Check sheet for the modelled part. Datum: model origin and axes. Units: mm. Face numbers are marked on the shaded views. Round coordinates to 2 decimals unless told otherwise and drop trailing zeros. Order: outer loops, then holes, each group sorted by start corner. A loop starts at its lowest first (then second) coordinate and runs counter-clockwise, first axis right, second up. Notation, with made-up numbers: (22.25, 29.25) -> (46.25, 29.25) arc R22 cw to (46.25, 52.25) -> close; hole circle Ø1 at (-40, 83.5). An arc over 180 degrees is marked (long way). Use CSV: the item, a comma, the result in double quotes.
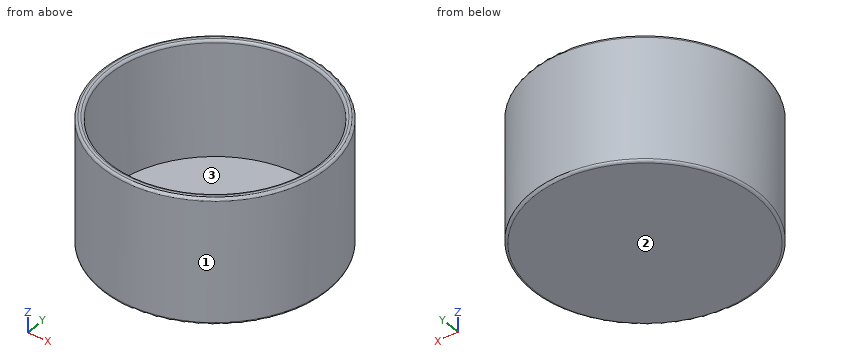
```python
from build123d import *

# Parameters (mm, degrees)
F0_R     = 57.15
F1_DEPTH = 5.08
F2_R     = 1.27
F5_E1_W  = 63.5
F5_E1_H  = 3.81
F7_R     = 1.26999
F8_R     = 1.27


# Not quite as in the source:
# - a fillet or chamfer is up to 0.001 mm smaller than in the source, because OpenCascade refuses the exact size


with BuildPart() as f1:
    # F0 (on Top) → F1 (new body)
    with BuildSketch(Plane.XY):
        Circle(F0_R)
    extrude(amount=F1_DEPTH)

    # F2
    f2_edges = [f1.edges().sort_by_distance(p)[0] for p in [
        (-57.15, 0, 0),
    ]]
    fillet(f2_edges, radius=F2_R)

    # F5_E1 (on explicit) → F6 (revolve)
    with BuildSketch(Plane(origin=(57.15, 0, 0), x_dir=(0, 0, 1), z_dir=(0, -1, 0))):
        with Locations((31.75, 1.905)):
            Rectangle(F5_E1_W, F5_E1_H)
    revolve(axis=Axis((0, 0, 5.08), (0, 0, 1)))

    # F7 (radius 1.27 in the source; OpenCascade refuses exactly that, so slightly less here)
    f7_edges = [f1.edges().sort_by_distance(p)[0] for p in [
        (-57.15, 0, 0),
    ]]
    fillet(f7_edges, radius=F7_R)

    # F8
    f8_edges = [f1.edges().sort_by_distance(p)[0] for p in [
        (-57.15, 0, 63.5),
        (-53.34, 0, 63.5),
    ]]
    fillet(f8_edges, radius=F8_R)


solid = f1.part
```
Q1. Mould release check, pull along Y, two halves, no side actions. Record for the marked faces 1, 2 and 3: pulls with the +Y half, pulls with the -Y half, needs draft (parallel to the pull), parting line crosses it, or undercut.
Result sheet:
face 1,"parting line crosses it"
face 2,"needs draft"
face 3,"undercut"
Q2. Sectioned sample at A-A, the plane y = 0. Enter the section's corners in (x, z), then the cut area to 3 significant figures.
Result sheet:
outline,"(-57.15, 1.27) arc R1.27 ccw to (-55.88, 0) -> (55.88, 0) arc R1.27 ccw to (57.15, 1.27) -> (57.15, 62.23) arc R1.27 ccw to (55.88, 63.5) -> (54.61, 63.5) arc R1.27 ccw to (53.34, 62.23) -> (53.34, 5.08) -> (-53.34, 5.08) -> (-53.34, 62.23) arc R1.27 ccw to (-54.61, 63.5) -> (-55.88, 63.5) arc R1.27 ccw to (-57.15, 62.23) -> close"
area,"1,020 mm^2"
Q3. Sectioned sample at C-C, the plane z = 44. Enter the section's corners in (x, y).
Result sheet:
outline,"circle Ø114.3 at (0, 0); hole circle Ø106.68 at (0, 0)"
Q4. Go/stop test with flat-tipped pins: pin 1 (1.5 mm diameter, centred on x = -15.5, z = 43, fed in from -Y); pin 2 (2 mm diameter, centred on y = 25.5, z = 55.5, fed in from -X); pin 3 (5 mm diameter, centred on x = 2.5, y = -26, fed in from -Z); pin 4 (12 mm diameter, centred on x = 44, z = 56, fed in from -Y). Record where each tip stops, or that it passes through.
Result sheet:
pin 1,"stops at y = -55.21"
pin 2,"stops at x = -51.63"
pin 3,"stops at z = 0"
pin 4,"stops at y = -42.69"
Q5. Scan lines: L1, parallel to Z at x = 28, y = 27; L2, parallel to Y at x = 0, z = 48; L3, parallel to X at y = -1, z = 37. Record each from-to range of solid material in increasing order.
Result sheet:
L1,"z = 0 to 5.08"
L2,"y = -57.15 to -53.34, 53.34 to 57.15"
L3,"x = -57.14 to -53.33, 53.33 to 57.14"
